Could you check a few things on this model? Use its own coordinates, in mm. Round coordinates to 2 decimals unless told otherwise and drop trailing zeros. Order: outer loops, then holes, each group sorted by start corner. A loop starts at its lowest first (then second) coordinate and runs counter-clockwise, first axis right, second up. Notation, with made-up numbers: (-13, 42.25) - (36, 42.25) arc R19 ccw to (36, 64.25) - close; hole circle Ø11 at (-20.5, 38.25). An arc over 180 degrees is marked (long way). Use one line per item in the form item = value.
from build123d import *

# Parameters (mm, degrees)
EXTRUDE_1_DEPTH     = 3
SKETCH_3_R          = 1.5
CUT_EXTRUDE_1_DEPTH = 65.101482042
FILLET_2_R          = 10
FILLET_3_R          = 10
CUT_EXTRUDE_3_DEPTH = 65.101482042


with BuildPart() as part:
    # 草图2 → 凸台-拉伸1 (new body)
    with BuildSketch(Plane.XY):
        Polygon((0, 0), (0, 15), (-30, 15), (-50, -25), (-50, -40), (-20, -40), align=None)
    extrude(amount=EXTRUDE_1_DEPTH)

    # 草图3 → 切除-拉伸1 (cut, through all)
    with BuildSketch(Plane.XY.offset(3)):
        with Locations((-5, 7.5)):
            Circle(SKETCH_3_R)
        with Locations((-25, 7.5)):
            Circle(SKETCH_3_R)
        with Locations((-45, -32.5)):
            Circle(SKETCH_3_R)
        with Locations((-25, -32.5)):
            Circle(SKETCH_3_R)
    extrude(amount=-CUT_EXTRUDE_1_DEPTH, mode=Mode.SUBTRACT)

    # 圆角2
    fillet_2_edges = [part.edges().sort_by_distance(p)[0] for p in [
        (-50, -25, 1.5),
        (0, 0, 1.5),
    ]]
    fillet(fillet_2_edges, radius=FILLET_2_R)

    # 圆角3
    fillet_3_edges = [part.edges().sort_by_distance(p)[0] for p in [
        (-50, -40, 1.5),
        (0, 15, 1.5),
    ]]
    fillet(fillet_3_edges, radius=FILLET_3_R)

    # 草图7 → 切除-拉伸3 (cut, through all)
    with BuildSketch(Plane.XY.offset(3)):
        with BuildLine():
            Line((-43.883436854, -22.829179607), (-32.883436854, -0.829179607))
            ThreePointArc((-32.883436854, -0.829179607), (-30.870975674, -0.158359214), (-30.200155281, -2.170820393))
            Line((-30.200155281, -2.170820393), (-41.200155281, -24.170820393))
            ThreePointArc((-41.200155281, -24.170820393), (-43.212616461, -24.841640786), (-43.883436854, -22.829179607))
        make_face()
        with BuildLine():
            Line((-29.700155281, -24.170820393), (-18.700155281, -2.170820393))
            ThreePointArc((-18.700155281, -2.170820393), (-19.370975674, -0.158359214), (-21.383436854, -0.829179607))
            Line((-21.383436854, -0.829179607), (-32.383436854, -22.829179607))
            ThreePointArc((-32.383436854, -22.829179607), (-31.712616461, -24.841640786), (-29.700155281, -24.170820393))
        make_face()
        with BuildLine():
            Line((-18.200155281, -24.170820393), (-7.200155281, -2.170820393))
            ThreePointArc((-7.200155281, -2.170820393), (-7.870975674, -0.158359214), (-9.883436854, -0.829179607))
            Line((-9.883436854, -0.829179607), (-20.883436854, -22.829179607))
            ThreePointArc((-20.883436854, -22.829179607), (-20.212616461, -24.841640786), (-18.200155281, -24.170820393))
        make_face()
    extrude(amount=-CUT_EXTRUDE_3_DEPTH, mode=Mode.SUBTRACT)


solid = part.part
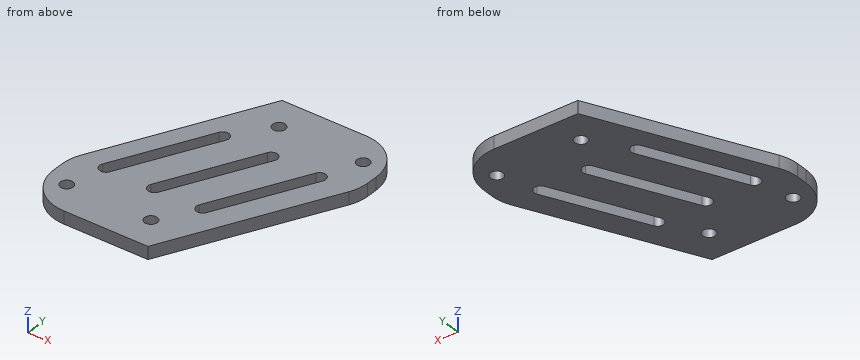
Item 1: Imagine slicing it at D-D on x = -25. Please give me the cut outline in (y, z), plus the area to 3 significant figures.
Found:
outline = (-40, 0) - (-34, 0) - (-34, 3) - (-40, 3) - close; (-31, 0) - (-14.77, 0) - (-14.77, 3) - (-31, 3) - close; (-8.06, 0) - (6, 0) - (6, 3) - (-8.06, 3) - close; (9, 0) - (15, 0) - (15, 3) - (9, 3) - close
area = 127 mm2
Item 2: Will this pin go through, and if not, where does the flat tip stop? P1, Ø1.8, axis at x = -25, y = 7.5, coming from the -Z side.
Found:
P1 = through
Item 3: Imagine slicing it at A-A on z = 1.45. Please give me the cut outline in (x, y), plus the area to 3 significant figures.
Found:
outline = (-50, -30) arc R10 ccw to (-40, -40) - (-20, -40) - (-1.06, -2.11) arc R10 ccw to (0, 2.36) - (0, 5) arc R10 ccw to (-10, 15) - (-30, 15) - (-48.94, -22.89) arc R10 ccw to (-50, -27.36) - close; hole circle Ø3 at (-45, -32.5); hole (-43.88, -22.83) arc R1.5 ccw to (-41.2, -24.17) - (-30.2, -2.17) arc R1.5 ccw to (-32.88, -0.83) - close; hole (-32.38, -22.83) arc R1.5 ccw to (-29.7, -24.17) - (-18.7, -2.17) arc R1.5 ccw to (-21.38, -0.83) - close; hole circle Ø3 at (-25, -32.5); hole circle Ø3 at (-25, 7.5); hole (-20.88, -22.83) arc R1.5 ccw to (-18.2, -24.17) - (-7.2, -2.17) arc R1.5 ccw to (-9.88, -0.83) - close; hole circle Ø3 at (-5, 7.5)
area = 1,640 mm2
Item 4: Imagine slicing it at C-C on y = -15.5. Please give me the cut outline in (x, z), plus the area to 3 significant figures.
Found:
outline = (-45.25, 0) - (-40.22, 0) - (-40.22, 3) - (-45.25, 3) - close; (-36.86, 0) - (-28.72, 0) - (-28.72, 3) - (-36.86, 3) - close; (-25.36, 0) - (-17.22, 0) - (-17.22, 3) - (-25.36, 3) - close; (-13.86, 0) - (-7.75, 0) - (-7.75, 3) - (-13.86, 3) - close
area = 82.3 mm2
Item 5: Imagine slicing it at B-B on x = -45. Please give me the cut outline in (y, z).
Found:
outline = (-38.66, 0) - (-34, 0) - (-34, 3) - (-38.66, 3) - close; (-31, 0) - (-15, 0) - (-15, 3) - (-31, 3) - close
Item 6: I need wall thicknesses on L1, parallel to Y at x = -25, z = 1.45; L2, parallel to X at y = -6.5, z = 0.95; L3, parallel to X at y = -20.5, z = 1.6. Which ranges of each line are inside material? Lowest first, please.
Found:
L1 = -40 to -34, -31 to -14.77, -8.06 to 6, 9 to 15
L2 = -40.75 to -35.72, -32.36 to -24.22, -20.86 to -12.72, -9.36 to -3.25
L3 = -47.75 to -42.72, -39.36 to -31.22, -27.86 to -19.72, -16.36 to -10.25
